Source: CAD feature listing. Evaluate the final solid. Frame: model axes, mm. A direction names the side the tool comes from. Round coordinates to 2 decimals unless told otherwise and drop trailing zeros. Loops run counter-clockwise (first coordinate to the right, second up) from the corner with the lowest first, then second, coordinate; pieces in that order, holes last. Notation, with made-up numbers: M 66.25,-24 L 109.25,-24 A25 cw 109.25,11 Z; hole C 22,29 d10. An arc over 180 degrees is marked long. Answer as a JSON object with one key per item and string values.
Autodesk Inventor part; units mm, degrees
ref_plane "YZ Plane" through (0, 0, 0) normal (1, 0, 0) x (0, 1, 0)
ref_plane "XZ Plane" through (0, 0, 0) normal (0, 1, 0) x (-1, 0, 0)
ref_plane "XY Plane" through (0, 0, 0) normal (0, 0, 1) x (1, 0, 0)
sketch "Sketch1" plane through (0, 0, 0) normal (0, 1, 0) x (-1, 0, 0)
  line L0 (63.5, 25.4) -> (-63.5, 25.4)
  line L1 (-63.5, 25.4) -> (-63.5, -25.4)
  line L2 (-63.5, -25.4) -> (63.5, -25.4)
  line L3 (63.5, -25.4) -> (63.5, 25.4)
  point P0 (0, 0)
  dimension "d0" = 50.8
  dimension "d1" = 25.4
  dimension "d2" = 63.5
  dimension "d3" = 127
extrude "Extrusion1" add sketch "Sketch1" along normal blind 6.35
sketch "Sketch2" plane through (0, 6.35, 0) normal (0, 1, 0) x (1, 0, 0)
  line L0 (-60.325, -22.225) -> (60.325, -22.225)
  line L1 (60.325, -22.225) -> (60.325, 22.225)
  line L2 (60.325, 22.225) -> (-60.325, 22.225)
  line L3 (-60.325, 22.225) -> (-60.325, -22.225)
  line L4 (-63.5, -25.4) -> (63.5, -25.4)
  line L5 (63.5, -25.4) -> (63.5, 25.4)
  line L6 (63.5, 25.4) -> (-63.5, 25.4)
  line L7 (-63.5, 25.4) -> (-63.5, -25.4)
  point P0 (0, 0)
  dimension "d6" = 3.175
  dimension "d7" = 3.175
  dimension "d8" = 3.175
  dimension "d9" = 3.175
extrude "Extrusion2" add sketch "Sketch2" along normal blind 38.1
fillet "Fillet1" radius 3.175 4 edges at (-60.325, 25.4, -22.225) (60.325, 25.4, -22.225) (60.325, 25.4, 22.225) (-60.325, 25.4, 22.225)
sketch "Sketch4" plane through (63.5, 0, -25.4) normal (0, 0, -1) x (-1, 0, 0)
  line L0 (127, 0) -> (127, 44.45)
  line L1 (127, 44.45) -> (104.775, 44.45)
  line L2 (104.775, 44.45) -> (104.775, 38.1)
  line L3 (104.775, 38.1) -> (127, 38.1)
  line L4 (127, 38.1) -> (127, 44.45)
  line L5 (74.6125, 44.45) -> (52.3875, 44.45)
  line L6 (52.3875, 44.45) -> (52.3875, 38.1)
  line L7 (52.3875, 38.1) -> (74.6125, 38.1)
  line L8 (74.6125, 38.1) -> (74.6125, 44.45)
  line L9 (22.225, 44.45) -> (0, 44.45)
  line L10 (0, 44.45) -> (0, 38.1)
  line L11 (0, 38.1) -> (22.225, 38.1)
  line L12 (22.225, 38.1) -> (22.225, 44.45)
  point P0 (63.5, 0)
  dimension "d28" = 22.225
  dimension "d29" = 6.35
  dimension "d32" = 52.3875
extrude "Extrusion4" [suppressed]
sketch "Sketch5" plane through (-63.5, 0, -25.4) normal (-1, 0, 0) x (0, 0, 1)
  line L0 (-15.24, 38.1) -> (0, 22.86)
  line L1 (0, 0) -> (0, 44.45)
  line L2 (0, 44.45) -> (0, 38.1)
  line L3 (0, 22.86) -> (0, 38.1)
  line L4 (0, 38.1) -> (-15.24, 38.1)
  point P0 (25.4, 0)
  dimension "d39" = 15.24
extrude "Extrusion5" [suppressed]
pattern_linear "Rectangular Pattern1" [suppressed]
pattern_linear "Rectangular Pattern2" [suppressed]
sketch "Sketch6" plane through (-60.325, 38.1, -40.64) normal (0, -1, 0) x (1, 0, 0)
  line L0 (123.825, 15.24) -> (-3.175, 15.24)
  line L1 (15.875, 0) -> (0, 0)
  line L2 (15.875, 0) -> (15.875, 15.24)
  line L3 (0, 15.24) -> (0, 0)
  point P0 (60.325, 40.64)
  point P1 (7.9375, 7.62)
  point P2 (60.3377, 7.62)
  point P3 (112.7379, 7.62)
  dimension "d48" = 7.62
  dimension "d49" = 15.24
  dimension "d50" = 15.875
  dimension "d51" = 7.9375
  dimension "d54" = 52.4002
hole "Hole1" [suppressed]
fillet "Fillet2" [suppressed]
fillet "Fillet3" [suppressed]
mirror "Mirror1" [suppressed]
fillet "Fillet4" [suppressed]
sketch "Sketch13" plane through (0, 44.45, 0) normal (0, 1, 0) x (1, 0, 0)
  line L0 (-74.295, 36.195) -> (74.295, 36.195)
  line L1 (74.295, 36.195) -> (74.295, -36.195)
  line L2 (74.295, -36.195) -> (-74.295, -36.195)
  line L3 (-74.295, -36.195) -> (-74.295, 36.195)
  line L4 (63.5, 25.4) -> (-63.5, 25.4)
  line L5 (-63.5, 25.4) -> (-63.5, -25.4)
  line L6 (-63.5, -25.4) -> (63.5, -25.4)
  line L7 (63.5, -25.4) -> (63.5, 25.4)
  point P0 (0, 0)
  dimension "d81" = 10.795
  dimension "d82" = 10.795
  dimension "d83" = 10.795
  dimension "d84" = 10.795
extrude "Extrusion12" add sketch "Sketch13" against normal blind 6.35
fillet "Fillet5" radius 3.175 8 edges at (63.5, 38.1, 0) (0, 38.1, -25.4) (-63.5, 38.1, 0) (0, 38.1, 25.4) (-74.295, 41.275, 36.195) (-74.295, 41.275, -36.195) (74.295, 41.275, 36.195) (74.295, 41.275, -36.195)
sketch "Sketch14" plane through (0, 38.1, 0) normal (0, -1, 0) x (1, 0, 0)
  line L0 (71.12, 36.195) -> (-71.12, 36.195)
  line L1 (66.675, 28.575) -> (-66.675, 28.575)
  line L2 (74.295, -33.02) -> (74.295, 33.02)
  line L3 (74.295, -33.02) -> (74.295, 33.02)
  line L4 (74.295, 0) -> (-74.2494, 0) construction
  line L5 (71.12, -36.195) -> (-71.12, -36.195)
  line L6 (66.675, -28.575) -> (66.675, 28.575)
  line L7 (-71.12, -36.195) -> (71.12, -36.195)
  line L8 (0, -36.195) -> (0, 36.195) construction
  point P0 (0, 0)
  point P1 (59.2667, 32.385)
  point P2 (44.45, 32.385)
  point P3 (29.6333, 32.385)
  point P4 (14.8167, 32.385)
  point P5 (0, 32.385)
  point P6 (-14.8167, 32.385)
  point P7 (-29.6333, 32.385)
  point P8 (-44.45, 32.385)
  point P9 (-59.2667, 32.385)
  point P10 (59.2667, -32.385)
  point P11 (44.45, -32.385)
  point P12 (29.6333, -32.385)
  point P13 (14.8167, -32.385)
  point P14 (0, -32.385)
  point P15 (-14.8167, -32.385)
  point P16 (-29.6333, -32.385)
  point P17 (-44.45, -32.385)
  point P18 (-59.2667, -32.385)
  point P19 (70.485, -27.1463)
  point P20 (70.485, -9.0488)
  point P21 (70.485, 9.0488)
  point P22 (70.485, 27.1463)
  point P23 (-70.485, -27.1462)
  point P24 (-70.485, -9.0487)
  point P25 (-70.485, 9.0488)
  point P26 (-70.485, 27.1463)
  dimension "d88" = 3.81
  dimension "d89" = 7.62
  dimension "d94" = 14.8167
  dimension "d99" = 118.5333
  dimension "d100" = 59.2667
  dimension "d101" = 7.62
  dimension "d102" = 3.81
  dimension "d103" = 9.0488
  dimension "d106" = 18.0975
  dimension "d111" = 54.2925
  dimension "d112" = 27.1462
hole "Hole2" at (59.2667, 38.1, 32.385) at (44.45, 38.1, 32.385) at (29.6333, 38.1, 32.385) at (14.8167, 38.1, 32.385) at (0, 38.1, 32.385) at (-14.8167, 38.1, 32.385) at (-29.6333, 38.1, 32.385) at (-44.45, 38.1, 32.385) at (-59.2667, 38.1, 32.385) at (-59.2667, 38.1, -32.385) at (-44.45, 38.1, -32.385) at (-29.6333, 38.1, -32.385) at (-14.8167, 38.1, -32.385) at (0, 38.1, -32.385) at (14.8167, 38.1, -32.385) at (29.6333, 38.1, -32.385) at (44.45, 38.1, -32.385) at (59.2667, 38.1, -32.385) at (70.485, 38.1, -27.1463) at (70.485, 38.1, -9.0488) at (70.485, 38.1, 9.0488) at (70.485, 38.1, 27.1463) at (-70.485, 38.1, -27.1462) at (-70.485, 38.1, -9.0487) at (-70.485, 38.1, 9.0488) at (-70.485, 38.1, 27.1463) direction (0, 1, 0) diameter 2.5146 depth 25.4 tip angle 118
sketch "Sketch17" plane through (0, 0, 0) normal (0, -1, 0) x (1, 0, 0)
  line L0 (50.4, -14.25) -> (43.6, -14.25)
  line L1 (43.6, -14.25) -> (43.6, 9.75)
  line L2 (43.6, 9.75) -> (50.4, 9.75)
  line L3 (50.4, 9.75) -> (50.4, -14.25)
  point P0 (0, 0)
extrude "Extrusion14" cut sketch "Sketch17" against normal blind 6.35
sketch "Sketch18" plane through (0, 0, 0) normal (0, -1, 0) x (1, 0, 0)
  line L0 (59.29, -7.85) -> (52.49, -7.85)
  line L1 (52.49, -7.85) -> (52.49, 5.95)
  line L2 (52.49, 5.95) -> (59.29, 5.95)
  line L3 (59.29, 5.95) -> (59.29, -7.85)
  line L4 (-56.75, -4.3) -> (-49.95, -4.3)
  line L5 (-49.95, -4.3) -> (-49.95, -14.2)
  line L6 (-49.95, -14.2) -> (-56.75, -14.2)
  line L7 (-56.75, -14.2) -> (-56.75, -4.3)
  point P0 (0, 0)
extrude "Extrusion15" cut sketch "Sketch18" against normal through all
sketch "Sketch19" plane through (0, 0, 0) normal (0, -1, 0) x (1, 0, 0)
  circle A0 centre (55.89, 8.15) radius 1.6
  circle A1 centre (55.89, -10.05) radius 1.6
  circle A2 centre (-53.35, -2.1) radius 1.6
  circle A3 centre (-53.35, -16.4) radius 1.6
  circle A4 centre (47, -16.4) radius 1.6
  circle A5 centre (47, 11.9) radius 1.6
  point P0 (0, 0)
extrude "Extrusion16" cut sketch "Sketch19" against normal through all
equation "\"d7\" = d6"
equation "\"d8\" = d6"
equation "\"d9\" = d6"
equation "\"d81\" = d83"
equation "\"d82\" = d83"
equation "\"d84\" = d83"
properties part number "Electronics Box" material "Aluminum 6061"
Item 1: Contact query for flat-ended pins moving along their axis: pin 1 Ø2 at (x, z) = (-29.63, 32.38) entering from +Y; pin 2 Ø10 at (x, y) = (-25.5, 10) entering from -Z; pin 3 Ø3 at (y, z) = (33, -14) entering from -X; pin 4 Ø12 at (x, z) = (25, -20.5) entering from +Y. Output: stop coordinate, or through.
Answer sheet:
{"pin 1": "passes through", "pin 2": "stops at z = -25.4", "pin 3": "stops at x = -63.5", "pin 4": "stops at y = 44.45"}
Item 2: Section A-A on z = -2.1. Return the cut outline in (x, y) (3 decimals), then the cut area to 3 significant figures.
Answer sheet:
{"outline": "M -74.295,38.1 L -66.675,38.1 A3.175 cw -63.5,34.925 L -63.5,0 L -54.95,0 L -54.95,6.35 L -60.325,6.35 L -60.325,44.45 L -74.295,44.45 Z; M -51.75,0 L 43.6,0 L 43.6,6.35 L -51.75,6.35 Z; M 50.4,0 L 52.49,0 L 52.49,6.35 L 50.4,6.35 Z; M 59.29,0 L 63.5,0 L 63.5,34.925 A3.175 cw 66.675,38.1 L 74.295,38.1 L 74.295,44.45 L 60.325,44.45 L 60.325,6.35 L 59.29,6.35 Z", "area": "1,080 mm²"}
Item 3: Section C-C on x = -53.35. Return the cut outline in (y, z) (3 decimals), then the cut area to 3 significant figures.
Answer sheet:
{"outline": "M 0,-25.4 L 34.925,-25.4 A3.175 cw 38.1,-28.575 L 38.1,-36.195 L 44.45,-36.195 L 44.45,-22.225 L 6.35,-22.225 L 6.35,-18 L 0,-18 Z; M 0,-14.8 L 6.35,-14.8 L 6.35,-14.2 L 0,-14.2 Z; M 0,-4.3 L 6.35,-4.3 L 6.35,-3.7 L 0,-3.7 Z; M 0,-0.5 L 6.35,-0.5 L 6.35,22.225 L 44.45,22.225 L 44.45,36.195 L 38.1,36.195 L 38.1,28.575 A3.175 cw 34.925,25.4 L 0,25.4 Z", "area": "602 mm²"}
Item 4: Section D-D on y = 3. Give the number of separate pieces and of enclosed holes in the cut face, then the cut area to 3 significant figures.
Answer sheet:
{"separate pieces": "1", "enclosed holes": "9", "area": "6,080 mm²"}
Item 5: Line query: probe 1 along Z at (x, y) = (55.89, 1.5); probe 2 along X at (y, z) = (4, 8); probe 3 along X at (y, z) = (41.5, 5.5) (3 decimals). Output: solid intervals per line, ascending. Write a range as from..to.
Answer sheet:
{"probe 1": "z = -25.4..-11.65, -8.45..-7.85, 5.95..6.55, 9.75..25.4", "probe 2": "x = -63.5..43.6, 50.4..54.3, 57.48..63.5", "probe 3": "x = -74.295..-60.325, 60.325..74.295"}
Item 6: Section B-B on z = -16.4. Return the cut outline in (x, y) (3 decimals).
Answer sheet:
{"outline": "M -74.295,38.1 L -66.675,38.1 A3.175 cw -63.5,34.925 L -63.5,0 L -54.95,0 L -54.95,6.35 L -60.325,6.35 L -60.325,44.45 L -74.295,44.45 Z; M -51.75,0 L 45.4,0 L 45.4,6.35 L -51.75,6.35 Z; M 48.6,0 L 63.5,0 L 63.5,34.925 A3.175 cw 66.675,38.1 L 74.295,38.1 L 74.295,44.45 L 60.325,44.45 L 60.325,6.35 L 48.6,6.35 Z"}
Item 7: Pull-direction query (Z, two-part tool) for faces 1 (the flat face through (-63.5, 17, 0)), 2 (the cylindrical face through (73.34, 41.23, -35.29)), 3 (the cylindrical face through (48.48, 3.13, -17.01)); classes: pulls with the +Z half, pulls with the -Z half, needs draft (parallel to the pull), parting line crosses it, or undercut.
Answer sheet:
{"face 1": "needs draft", "face 2": "pulls with the -Z half", "face 3": "undercut"}
Item 8: Access query for faces 4 (the cylindrical face through (64.41, 37.15, -0.4)), 5 (the flat face through (56, 3, -7.85)), 6 (the flat face through (1, 6.35, 0)). Directions: +Z, -Z, +X, -X, +Y, -Y. A direction counts if a zero-diameter tool reaches every point of the face in a straight line with its end or side. Return the directions, or none.
Answer sheet:
{"face 4": "+Z, -Z, +X, -Y", "face 5": "+Y, -Y", "face 6": "+Y"}
